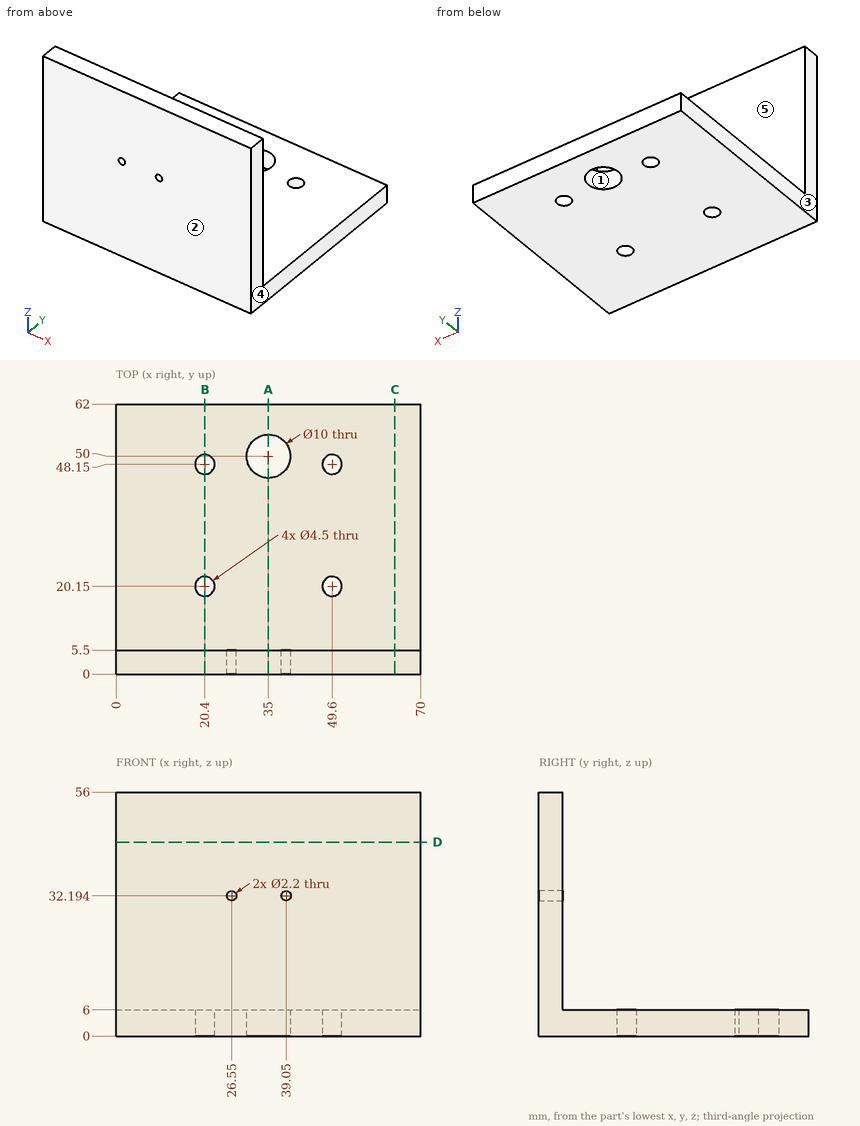
Job drawing, mm, ordinate dimensions from the low corner. One solid piece. A direction names the side the tool comes from. Give positions to 0.01 mm unless a question says otherwise; leave off trailing zeros. Write each loop counter-clockwise with the first axis right and the second up, starting at its lowest first coordinate (ties: lowest second). Pieces come first, ordered by that corner, then holes. Notation, with made-up numbers: M 65.5,-24 L 79.5,-24 A25 ccw 79.5,10 Z; hole C 69,70.5 d10. An arc over 180 degrees is marked long. One line per item, written item: value. Start each with the question number.
Q1. Saw through at C-C, the plane x = 64. Write the cut outline in (y, z).
Q2. Probe probe 1 along X at (y, z) = (20, 3) (1 decimal); probe 2 along Y at (x, z) = (20.4, 4.15); probe 3 along Y at (x, z) = (35, 1.85). List the from-to ranges inside material, lowest first. Write a range as [from, to].
Q3. Saw through at D-D, the plane z = 44.5. Write the cut outline in (x, y).
Q4. 3-axis set-ups, long thin cutter, end or side, ignore diameter. For the marked faces 4 and 5: which of +Z, -Z, +X, -X, +Y, -Y reach the whole face in a straight line?
Q5. Two-plate mould, pull along X, no slides. Class the marked faces 1, 2 and 3: +X half, -X half, draft (parallel to the pull), parting line (faces both ways), or undercut.
Q6. Saw through at B-B, the plane x = 20.4. Write the cut outline in (y, z).
Q7. Saw through at A-A, the plane x = 35. Write the cut outline in (y, z), plus the area to 3 significant figures.
Q8. Drop flat-ended pins along their axis: pin 1 Ø25 at (x, z) = (43.5, 28) entering from +Y; pin 2 Ø12 at (x, y) = (56.5, 52) entering from +Z; pin 3 Ø3.5 at (x, y) = (49.6, 20.15) entering from -Z. Give the stop position or say it passes through.
Output values:
1. outline: M 0,0 L 62,0 L 62,6 L 5.5,6 L 5.5,56 L 0,56 Z
2. probe 1: x = [0, 18.2], [22.6, 47.4], [51.8, 70]
2. probe 2: y = [0, 17.9], [22.4, 45.9], [50.4, 62]
2. probe 3: y = [0, 45], [55, 62]
3. outline: M 0,0 L 70,0 L 70,5.5 L 0,5.5 Z
4. face 4: +Z, -Z, +X, +Y, -Y
4. face 5: +Z, +X, -X, +Y
5. face 1: undercut
5. face 2: draft
5. face 3: -X half
6. outline: M 0,0 L 17.9,0 L 17.9,6 L 5.5,6 L 5.5,56 L 0,56 Z; M 22.4,0 L 45.9,0 L 45.9,6 L 22.4,6 Z; M 50.4,0 L 62,0 L 62,6 L 50.4,6 Z
7. outline: M 0,0 L 45,0 L 45,6 L 5.5,6 L 5.5,56 L 0,56 Z; M 55,0 L 62,0 L 62,6 L 55,6 Z
7. area: 587 mm²
8. pin 1: stops at y = 5.5
8. pin 2: stops at z = 6
8. pin 3: passes through
